Source: CAD feature listing. Evaluate the final solid. Frame: model axes, mm. Round coordinates to 2 decimals unless told otherwise and drop trailing zeros. Loops run counter-clockwise (first coordinate to the right, second up) from the corner with the lowest first, then second, coordinate; pieces in that order, holes last. Notation, with made-up numbers: (-24, 41.25) - (-16, 41.25) arc R17 cw to (-16, 71.25) - close; hole circle Ø3 at (1.5, 74). An arc over 180 degrees is marked (long way). One line per question, with ' | ' between items. Start each with the question number.
1. Cut plane A-A (z = 71). Return loops of the section in (x, y).
2. Ray query, line 1 (Y direction, x = -7.25, z = 145); line 2 (Y direction, x = -3, z = 181). Return the intervals inside material, ascending.
3. Cut plane B-B (x = 1.5). Return loops of the section in (y, z), then the cut area to 3 significant figures.
4. Pin query (flat end, axial travel): pin 1 (6.5 mm diameter, centred on x = 0.5, z = 125, fed in from -Y); pin 2 (1 mm diameter, centred on x = 0, z = 119, fed in from +Y); pin 3 (4 mm diameter, centred on y = 0.5, z = 67.5, fed in from +X). Return the tip coordinate at first contact, or that it passes through.
Autodesk Inventor part; units mm, degrees
ref_plane "YZ Plane" through (0, 0, 0) normal (1, 0, 0) x (0, 1, 0)
ref_plane "XZ Plane" through (0, 0, 0) normal (0, 1, 0) x (-1, 0, 0)
ref_plane "XY Plane" through (0, 0, 0) normal (0, 0, 1) x (1, 0, 0)
sketch "Sketch1" plane through (0, 0, 0) normal (0, 0, 1) x (1, 0, 0)
  line L0 (10, -10) -> (-10, 10) construction
  line L1 (-10, -10) -> (10, 10) construction
  line L2 (-4, 6) -> (4, 6)
  line L3 (4, 6) -> (4, 14)
  line L4 (4, 14) -> (-4, 14)
  line L5 (-4, 14) -> (-4, 6)
  line L6 (-4, 6) -> (4, 14) construction
  line L7 (4, 6) -> (-4, 14) construction
  line L8 (14, -4) -> (6, -4)
  line L9 (6, -4) -> (6, 4)
  line L10 (6, 4) -> (14, 4)
  line L11 (14, 4) -> (14, -4)
  line L12 (14, -4) -> (6, 4) construction
  line L13 (6, -4) -> (14, 4) construction
  line L14 (-4, -6) -> (4, -6)
  line L15 (4, -6) -> (4, -14)
  line L16 (4, -14) -> (-4, -14)
  line L17 (-4, -14) -> (-4, -6)
  line L18 (-4, -6) -> (4, -14) construction
  line L19 (4, -6) -> (-4, -14) construction
  line L20 (-14, 4) -> (-6, 4)
  line L21 (-6, 4) -> (-6, -4)
  line L22 (-6, -4) -> (-14, -4)
  line L23 (-14, -4) -> (-14, 4)
  line L24 (-14, 4) -> (-6, -4) construction
  line L25 (-6, 4) -> (-14, -4) construction
  line L26 (-10, -10) -> (-10, 0)
  line L27 (-10, 4) -> (-10, 10)
  line L28 (-10, 10) -> (0, 10)
  line L29 (4, 10) -> (10, 10)
  line L30 (10, 10) -> (10, 4)
  line L31 (10, 0) -> (10, -10)
  line L32 (10, -10) -> (4, -10)
  line L33 (0, -10) -> (-10, -10)
  point P0 (0, 0)
  point P1 (-4, 10)
  point P2 (10, -4)
  point P3 (-4, -10)
  point P4 (-10, -4)
  dimension "d0" = 20
  dimension "d1" = 20
  dimension "d2" = 8
  dimension "d3" = 8
  dimension "d4" = 8
  dimension "d5" = 8
  dimension "d6" = 8
  dimension "d7" = 8
  dimension "d8" = 8
  dimension "d9" = 8
extrude "Extrusion1" add sketch "Sketch1" along normal blind 250 contours L2 L3 L29 L30 L10 L9 L8 L31 L32 L15 L14 L17 L33 L26 L22 L21 L20 L27 L28 L5
ref_plane "Work Plane1" through (4, 0, 0) normal (0, 1, 0) x (1, 0, 0)
ref_plane "Work Plane2" through (0, -10, 0) normal (1, 0, 0) x (0, 0, -1)
properties part number "Neje_Base_Rod_20mm"
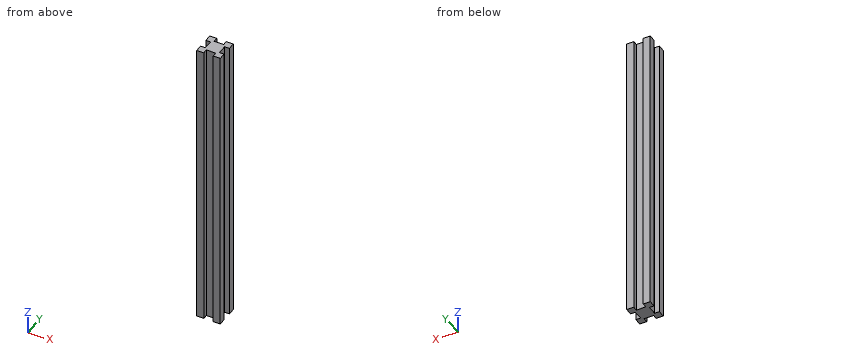
Answers follow:
1) outline: (-10, -10) - (-4, -10) - (-4, -6) - (4, -6) - (4, -10) - (10, -10) - (10, -4) - (6, -4) - (6, 4) - (10, 4) - (10, 10) - (4, 10) - (4, 6) - (-4, 6) - (-4, 10) - (-10, 10) - (-10, 4) - (-6, 4) - (-6, -4) - (-10, -4) - close
2) line 1: y = -10 to -4, 4 to 10 | line 2: y = -6 to 6
3) outline: (-6, 0) - (6, 0) - (6, 250) - (-6, 250) - close | area: 3,000 mm2
4) pin 1: stops at y = -6 | pin 2: stops at y = 6 | pin 3: stops at x = 6
